from build123d import *

# Parameters (mm, degrees)
SKETCH1_W           = 92.6
SKETCH1_H           = 300
BOSS_EXTRUDE1_DEPTH = 2
SKETCH3_R           = 2.25
SKETCH3_W           = 8.48
SKETCH3_H           = 51.5
SKETCH3_H_2         = 50
SKETCH3_H_3         = 53
CUT_EXTRUDE2_DEPTH  = 10
FILLET1_R           = 2
SKETCH4_R           = 1.85
CUT_EXTRUDE3_DEPTH  = 5
SKETCH5_R           = 1.85
CUT_EXTRUDE4_DEPTH  = 10
SKETCH6_R           = 1.85
CUT_EXTRUDE5_DEPTH  = 8.5
CUT_EXTRUDE6_DEPTH  = 8.5


with BuildPart() as part:
    # Sketch1 → Boss-Extrude1 (new body)
    with BuildSketch(Plane.XY):
        Rectangle(SKETCH1_W, SKETCH1_H)
    extrude(amount=BOSS_EXTRUDE1_DEPTH)

    # Sketch3 → Cut-Extrude2 (cut)
    with BuildSketch(Plane.XY):
        with Locations((-42.06, 75)):
            Circle(SKETCH3_R)
        with Locations((42.06, 125)):
            Circle(SKETCH3_R)
        with Locations((42.06, 25)):
            Circle(SKETCH3_R)
        with Locations((42.06, -75)):
            Circle(SKETCH3_R)
        with Locations((-42.06, -25)):
            Circle(SKETCH3_R)
        with Locations((-42.06, -125)):
            Circle(SKETCH3_R)
        with Locations((-42.06, 124.25)):
            Rectangle(SKETCH3_W, SKETCH3_H)
        with Locations((42.06, 75)):
            Rectangle(SKETCH3_W, SKETCH3_H_2)
        with Locations((42.06, -25)):
            Rectangle(SKETCH3_W, SKETCH3_H_2)
        with Locations((-42.06, 25)):
            Rectangle(SKETCH3_W, SKETCH3_H_3)
        with Locations((-42.06, -75)):
            Rectangle(SKETCH3_W, SKETCH3_H_3)
        with Locations((42.06, -125)):
            Rectangle(SKETCH3_W, SKETCH3_H_2)
    extrude(amount=CUT_EXTRUDE2_DEPTH, mode=Mode.SUBTRACT)

    # Fillet1
    fillet1_edges = [part.edges().sort_by_distance(p)[0] for p in [
        (46.3, -100, 1),
        (37.82, -100, 1),
        (37.82, -150, 1),
        (46.3, 50, 1),
        (46.3, 100, 1),
        (37.82, 100, 1),
        (37.82, 50, 1),
        (-46.3, -48.5, 1),
        (-46.3, -101.5, 1),
        (-37.82, -101.5, 1),
        (-37.82, -48.5, 1),
        (37.82, 0, 1),
        (37.82, -50, 1),
        (46.3, -50, 1),
        (46.3, 0, 1),
        (46.3, 150, 1),
        (-46.3, -150, 1),
        (-46.3, 51.5, 1),
        (-46.3, -1.5, 1),
        (-37.82, -1.5, 1),
        (-37.82, 51.5, 1),
        (-46.3, 98.5, 1),
        (-37.82, 98.5, 1),
        (-37.82, 150, 1),
    ]]
    fillet(fillet1_edges, radius=FILLET1_R)

    # Sketch4 → Cut-Extrude3 (cut)
    with BuildSketch(Plane(origin=(0, 0, 0), x_dir=(-1, 0, 0), z_dir=(0, 0, -1))):
        with Locations((-8.125, -79)):
            Circle(SKETCH4_R)
        with Locations((8.125, -48.8)):
            Circle(SKETCH4_R)
    extrude(amount=-CUT_EXTRUDE3_DEPTH, mode=Mode.SUBTRACT)

    # Sketch5 → Cut-Extrude4 (cut)
    with BuildSketch(Plane(origin=(0, 0, 0), x_dir=(-1, 0, 0), z_dir=(0, 0, -1))):
        with Locations((-15, -13)):
            Circle(SKETCH5_R)
        with Locations((15, -13)):
            Circle(SKETCH5_R)
        with BuildLine():
            Line((20.6, 3.5), (35.6, 3.5))
            ThreePointArc((35.6, 3.5), (36.307106781, 3.207106781), (36.6, 2.5))
            Line((36.6, 2.5), (36.6, -18.5))
            ThreePointArc((36.6, -18.5), (36.307106781, -19.207106781), (35.6, -19.5))
            Line((35.6, -19.5), (20.6, -19.5))
            ThreePointArc((20.6, -19.5), (19.892893219, -19.207106781), (19.6, -18.5))
            Line((19.6, -18.5), (19.6, 2.5))
            ThreePointArc((19.6, 2.5), (19.892893219, 3.207106781), (20.6, 3.5))
        make_face()
        with BuildLine():
            Line((-35.6, 3.588199514), (-20.6, 3.588199514))
            ThreePointArc((-20.6, 3.588199514), (-19.892893219, 3.295306295), (-19.6, 2.588199514))
            Line((-19.6, 2.588199514), (-19.6, -18.411800486))
            ThreePointArc((-19.6, -18.411800486), (-19.892893219, -19.118907267), (-20.6, -19.411800486))
            Line((-20.6, -19.411800486), (-35.6, -19.411800486))
            ThreePointArc((-35.6, -19.411800486), (-36.307106781, -19.118907267), (-36.6, -18.411800486))
            Line((-36.6, -18.411800486), (-36.6, 2.588199514))
            ThreePointArc((-36.6, 2.588199514), (-36.307106781, 3.295306295), (-35.6, 3.588199514))
        make_face()
    extrude(amount=-CUT_EXTRUDE4_DEPTH, mode=Mode.SUBTRACT)

    # Sketch6 → Cut-Extrude5 (cut)
    with BuildSketch(Plane(origin=(0, 0, 0), x_dir=(-1, 0, 0), z_dir=(0, 0, -1))):
        with Locations((-16.5, 74.5)):
            Circle(SKETCH6_R)
        with Locations((16.5, 74.5)):
            Circle(SKETCH6_R)
        with Locations((16.5, 54.5)):
            Circle(SKETCH6_R)
        with Locations((-16.5, 54.5)):
            Circle(SKETCH6_R)
    extrude(amount=-CUT_EXTRUDE5_DEPTH, mode=Mode.SUBTRACT)

    # Sketch7 → Cut-Extrude6 (cut)
    with BuildSketch(Plane(origin=(0, 0, 0), x_dir=(-1, 0, 0), z_dir=(0, 0, -1))):
        with BuildLine():
            Line((25, 93), (-25, 93))
            ThreePointArc((-25, 93), (-28.535533906, 94.464466094), (-30, 98))
            Line((-30, 98), (-30, 138))
            ThreePointArc((-30, 138), (-28.535533906, 141.535533906), (-25, 143))
            Line((-25, 143), (25, 143))
            ThreePointArc((25, 143), (28.535533906, 141.535533906), (30, 138))
            Line((30, 138), (30, 98))
            ThreePointArc((30, 98), (28.535533906, 94.464466094), (25, 93))
        make_face()
        with BuildLine():
            Line((25, -143), (-25, -143))
            ThreePointArc((-25, -143), (-28.535533906, -141.535533906), (-30, -138))
            Line((-30, -138), (-30, -98))
            ThreePointArc((-30, -98), (-28.535533906, -94.464466094), (-25, -93))
            Line((-25, -93), (25, -93))
            ThreePointArc((25, -93), (28.535533906, -94.464466094), (30, -98))
            Line((30, -98), (30, -138))
            ThreePointArc((30, -138), (28.535533906, -141.535533906), (25, -143))
        make_face()
    extrude(amount=-CUT_EXTRUDE6_DEPTH, mode=Mode.SUBTRACT)


solid = part.part
Source: CAD feature listing. Evaluate the final solid. Frame: model axes, mm. A direction names the side the tool comes from. Give positions to 0.01 mm unless a question says otherwise; leave off trailing zeros. Order: outer loops, then holes, each group sorted by start corner. A loop starts at its lowest first (then second) coordinate and runs counter-clockwise, first axis right, second up. Notation, with made-up numbers: (30, 24.5) -> (83, 24.5) arc R24 cw to (83, 60.5) -> close; hole circle Ø10 at (62, 24.25). An arc over 180 degrees is marked (long way). Use a Markdown table: item, result.
1) Section query B-B, the plane z = 1.65. Count the separate pieces of the cut face and the enclosed holes in it, then the cut area to 3 significant figures.
Answer list:
| item | result |
|---|---|
| separate pieces | 1 |
| enclosed holes | 18 |
| area | 18,300 mm² |
2) Ray query, line 1 along Y through (x, z) = (42.06, 1.05); line 2 along Y through (x, z) = (18.5, 0.25); line 3 along Y through (x, z) = (-42.06, 0.9). Return the intervals inside material, ascending. Write a range as [from, to].
Answer list:
| item | result |
|---|---|
| line 1 | [-100, -77.25], [-72.75, -50], [0, 22.75], [27.25, 50], [100, 122.75], [127.25, 150] |
| line 2 | [-150, -143], [-93, 93], [143, 150] |
| line 3 | [-150, -127.25], [-122.75, -101.5], [-48.5, -27.25], [-22.75, -1.5], [51.5, 72.75], [77.25, 98.5] |
3) Section query A-A, the plane y = -64.5. Return the cut outline in (x, z).
Answer list:
| item | result |
|---|---|
| outline | (-37.82, 0) -> (46.3, 0) -> (46.3, 2) -> (-37.82, 2) -> close |
4) Contact query for flat-ended pins moving along their axis: P1, Ø6, axis at x = -16.5, y = 74.5, coming from the -Z side; P2, Ø0.6, axis at y = -2.5, z = 0.5, coming from the +X side; P3, Ø0.6, axis at y = 120.5, z = 1, coming from the -X side. Output: stop coordinate, or through.
Answer list:
| item | result |
|---|---|
| P1 | z = 0 |
| P2 | x = 37.82 |
| P3 | x = -37.82 |
5) Mould query, pull axis Y, two halves, no side actions, for faces 1 (the cylindrical face through (-28, -94, 1)), 2 (the flat face through (-1, 2, 2)), 3 (the cylindrical face through (-28, 142, 1)). Classes: +Y half, -Y half, draft (parallel to the pull), parting line (faces both ways), or undercut.
Answer list:
| item | result |
|---|---|
| face 1 | undercut |
| face 2 | draft |
| face 3 | undercut |
6) Reachability of faces 4 (the flat face through (-1, 2, 0)), 5 (the cylindrical face through (28, 94, 1)) from +Z, -Z, +X, -X, +Y, -Y: full face, straight path, thin tool, end or side. Return the list, or none.
Answer list:
| item | result |
|---|---|
| face 4 | -Z, +X, -X, +Y, -Y |
| face 5 | +Z, -Z |
